Input: part model. Units: mm. Frame: model coordinates. A direction names the side the tool comes from. Give positions to 0.01 mm unless a question says otherwise; leave off trailing zeros. Loops run counter-clockwise (first coordinate to the right, second up) from the corner with the lowest first, then second, coordinate; pieces in that order, holes last. Notation, with made-up numbers: (-36, 46.5) - (-1, 46.5) arc R19 cw to (-1, 72.5) - close; hole circle Ø2 at (76.5, -38). An arc over 180 degrees is marked (long way). One line per item, written item: value.
from build123d import *

# Parameters (mm, degrees)
F0_R     = 63.5
F0_R_2   = 57.15
F0_R_3   = 1.3462
F1_DEPTH = 6.35
F2_START = 3.175
F2_DEPTH = 3.175
F3_SIZE  = 0.635
F4_DEPTH = 1.27


with BuildPart() as f1:
    # F0 (on Top) → F1 (new body)
    with BuildSketch(Plane.XY):
        Circle(F0_R)
        Circle(F0_R_2, mode=Mode.SUBTRACT)
        Circle(F0_R_2)
        with Locations((6.0491874454, -10.4775)):
            Circle(F0_R_3, mode=Mode.SUBTRACT)
        with BuildLine():
            ThreePointArc((-41.4540905122, -2.3213766309), (-39.8240691544, -4.0494939415), (-39.2315905122, -6.35))
            ThreePointArc((-39.2315905122, -6.35), (-46.2945965707, -10.5200213579), (-46.5340905122, -2.3213766309))
            Line((-46.5340905122, -2.3213766309), (-46.5340905122, 2.3213766309))
            ThreePointArc((-46.5340905122, 2.3213766309), (-46.2945965707, 10.5200213579), (-39.2315905122, 6.35))
            ThreePointArc((-39.2315905122, 6.35), (-39.8240691544, 4.0494939415), (-41.4540905122, 2.3213766309))
            Line((-41.4540905122, 2.3213766309), (-41.4540905122, -2.3213766309))
        make_face(mode=Mode.SUBTRACT)
        with Locations((-12.0983748909, 0)):
            Circle(F0_R_3, mode=Mode.SUBTRACT)
        with Locations((6.0491874454, 10.4775)):
            Circle(F0_R_3, mode=Mode.SUBTRACT)
        with BuildLine():
            ThreePointArc((48.7565905122, 6.35), (48.1641118701, 4.0494939415), (46.5340905122, 2.3213766309))
            Line((46.5340905122, 2.3213766309), (46.5340905122, -2.3213766309))
            ThreePointArc((46.5340905122, -2.3213766309), (48.1641118701, -4.0494939415), (48.7565905122, -6.35))
            ThreePointArc((48.7565905122, -6.35), (41.6935844538, -10.5200213579), (41.4540905122, -2.3213766309))
            Line((41.4540905122, -2.3213766309), (41.4540905122, 2.3213766309))
            ThreePointArc((41.4540905122, 2.3213766309), (41.6935844538, 10.5200213579), (48.7565905122, 6.35))
        make_face(mode=Mode.SUBTRACT)
        with BuildLine():
            ThreePointArc((-46.5340905122, -2.3213766309), (-46.2945965707, -10.5200213579), (-39.2315905122, -6.35))
            ThreePointArc((-39.2315905122, -6.35), (-39.8240691544, -4.0494939415), (-41.4540905122, -2.3213766309))
            Line((-41.4540905122, -2.3213766309), (-41.4540905122, -6.35))
            ThreePointArc((-41.4540905122, -6.35), (-43.9940905122, -8.89), (-46.5340905122, -6.35))
            Line((-46.5340905122, -6.35), (-46.5340905122, -2.3213766309))
        make_face()
        with BuildLine():
            ThreePointArc((41.4540905122, 6.35), (43.9940905122, 8.89), (46.5340905122, 6.35))
            Line((46.5340905122, 6.35), (46.5340905122, 2.3213766309))
            ThreePointArc((46.5340905122, 2.3213766309), (48.1641118701, 4.0494939415), (48.7565905122, 6.35))
            ThreePointArc((48.7565905122, 6.35), (41.6935844538, 10.5200213579), (41.4540905122, 2.3213766309))
            Line((41.4540905122, 2.3213766309), (41.4540905122, 6.35))
        make_face()
    extrude(amount=F1_DEPTH)

    # F0 (on Top) → F2 (cut)
    with BuildSketch(Plane.XY.offset(F2_START)):
        with BuildLine():
            ThreePointArc((-46.5340905122, -2.3213766309), (-46.2945965707, -10.5200213579), (-39.2315905122, -6.35))
            ThreePointArc((-39.2315905122, -6.35), (-39.8240691544, -4.0494939415), (-41.4540905122, -2.3213766309))
            Line((-41.4540905122, -2.3213766309), (-41.4540905122, -6.35))
            ThreePointArc((-41.4540905122, -6.35), (-43.9940905122, -8.89), (-46.5340905122, -6.35))
            Line((-46.5340905122, -6.35), (-46.5340905122, -2.3213766309))
        make_face()
        with BuildLine():
            Line((-41.4540905122, -6.35), (-41.4540905122, -2.3213766309))
            ThreePointArc((-41.4540905122, -2.3213766309), (-43.9940905122, -1.5875), (-46.5340905122, -2.3213766309))
            Line((-46.5340905122, -2.3213766309), (-46.5340905122, -6.35))
            ThreePointArc((-46.5340905122, -6.35), (-43.9940905122, -3.81), (-41.4540905122, -6.35))
        make_face()
        with BuildLine():
            Line((46.5340905122, 2.3213766309), (46.5340905122, 6.35))
            ThreePointArc((46.5340905122, 6.35), (43.9940905122, 3.81), (41.4540905122, 6.35))
            Line((41.4540905122, 6.35), (41.4540905122, 2.3213766309))
            ThreePointArc((41.4540905122, 2.3213766309), (43.9940905122, 1.5875), (46.5340905122, 2.3213766309))
        make_face()
        with BuildLine():
            ThreePointArc((41.4540905122, 6.35), (43.9940905122, 8.89), (46.5340905122, 6.35))
            Line((46.5340905122, 6.35), (46.5340905122, 2.3213766309))
            ThreePointArc((46.5340905122, 2.3213766309), (48.1641118701, 4.0494939415), (48.7565905122, 6.35))
            ThreePointArc((48.7565905122, 6.35), (41.6935844538, 10.5200213579), (41.4540905122, 2.3213766309))
            Line((41.4540905122, 2.3213766309), (41.4540905122, 6.35))
        make_face()
    extrude(amount=F2_DEPTH, mode=Mode.SUBTRACT)

    # F3
    f3_edges = [f1.edges().sort_by_distance(p)[0] for p in [
        (-63.5, 0, 6.35),
    ]]
    chamfer(f3_edges, length=F3_SIZE)

    # F0 (on Top) → F4 (cut)
    with BuildSketch(Plane.XY):
        Circle(F0_R_2)
        with Locations((6.0491874454, -10.4775)):
            Circle(F0_R_3, mode=Mode.SUBTRACT)
        with BuildLine():
            ThreePointArc((-41.4540905122, -2.3213766309), (-39.8240691544, -4.0494939415), (-39.2315905122, -6.35))
            ThreePointArc((-39.2315905122, -6.35), (-46.2945965707, -10.5200213579), (-46.5340905122, -2.3213766309))
            Line((-46.5340905122, -2.3213766309), (-46.5340905122, 2.3213766309))
            ThreePointArc((-46.5340905122, 2.3213766309), (-46.2945965707, 10.5200213579), (-39.2315905122, 6.35))
            ThreePointArc((-39.2315905122, 6.35), (-39.8240691544, 4.0494939415), (-41.4540905122, 2.3213766309))
            Line((-41.4540905122, 2.3213766309), (-41.4540905122, -2.3213766309))
        make_face(mode=Mode.SUBTRACT)
        with Locations((-12.0983748909, 0)):
            Circle(F0_R_3, mode=Mode.SUBTRACT)
        with Locations((6.0491874454, 10.4775)):
            Circle(F0_R_3, mode=Mode.SUBTRACT)
        with BuildLine():
            ThreePointArc((48.7565905122, 6.35), (48.1641118701, 4.0494939415), (46.5340905122, 2.3213766309))
            Line((46.5340905122, 2.3213766309), (46.5340905122, -2.3213766309))
            ThreePointArc((46.5340905122, -2.3213766309), (48.1641118701, -4.0494939415), (48.7565905122, -6.35))
            ThreePointArc((48.7565905122, -6.35), (41.6935844538, -10.5200213579), (41.4540905122, -2.3213766309))
            Line((41.4540905122, -2.3213766309), (41.4540905122, 2.3213766309))
            ThreePointArc((41.4540905122, 2.3213766309), (41.6935844538, 10.5200213579), (48.7565905122, 6.35))
        make_face(mode=Mode.SUBTRACT)
        with BuildLine():
            ThreePointArc((-46.5340905122, -2.3213766309), (-46.2945965707, -10.5200213579), (-39.2315905122, -6.35))
            ThreePointArc((-39.2315905122, -6.35), (-39.8240691544, -4.0494939415), (-41.4540905122, -2.3213766309))
            Line((-41.4540905122, -2.3213766309), (-41.4540905122, -6.35))
            ThreePointArc((-41.4540905122, -6.35), (-43.9940905122, -8.89), (-46.5340905122, -6.35))
            Line((-46.5340905122, -6.35), (-46.5340905122, -2.3213766309))
        make_face()
        with BuildLine():
            ThreePointArc((41.4540905122, 6.35), (43.9940905122, 8.89), (46.5340905122, 6.35))
            Line((46.5340905122, 6.35), (46.5340905122, 2.3213766309))
            ThreePointArc((46.5340905122, 2.3213766309), (48.1641118701, 4.0494939415), (48.7565905122, 6.35))
            ThreePointArc((48.7565905122, 6.35), (41.6935844538, 10.5200213579), (41.4540905122, 2.3213766309))
            Line((41.4540905122, 2.3213766309), (41.4540905122, 6.35))
        make_face()
    extrude(amount=F4_DEPTH, mode=Mode.SUBTRACT)


solid = f1.part
Item 1: Section A-A, the plane x = 0. Output: boundary loops of the cut face in (y, z) (3 decimals), and give its area (3 significant figures).
Verdict:
outline: (-63.5, 0) - (-57.15, 0) - (-57.15, 1.27) - (57.15, 1.27) - (57.15, 0) - (63.5, 0) - (63.5, 5.715) - (62.865, 6.35) - (-62.865, 6.35) - (-63.5, 5.715) - close
area: 661 mm^2
Item 2: Material intervals for L1, parallel to X at y = -9, z = 5.25; L2, parallel to Z at x = -12.5, y = -2.5; L3, parallel to X at y = 3, z = 4.5, sorted ascending.
Verdict:
L1: x = -62.86 to -47.95, -40.04 to 40.04, 47.95 to 62.86
L2: z = 1.27 to 6.35
L3: x = -63.43 to -47.38, -40.61 to 40.61, 47.38 to 63.43
Item 3: Access query for faces 4 (the face through (-57.095, 2.513, 0.626)), 5 (the face through (-44, -10, 3.175)), 6 (the face through (46.534, 1, 3)). Directions: +Z, -Z, +X, -X, +Y, -Y. A direction counts if a zero-diameter tool reaches every point of the face in a straight line with its end or side. Return the directions, or none.
Verdict:
face 4: -Z
face 5: +Z
face 6: +Z, -Z
Item 4: Section B-B, the plane z = 4.75. Count the separate pieces of the cut face and the enclosed holes in it, and give its area (3 significant figures).
Verdict:
separate pieces: 1
enclosed holes: 5
area: 12,300 mm^2
Item 5: Pin query (flat end, axial travel): P1, Ø2, axis at x = -12.1, y = 0, coming from the +Z side; P2, Ø3, axis at y = 21, z = 4.5, coming from the -X side; P3, Ø5.5, axis at x = -43.99, y = -6.35, coming from the +Z side (3 decimals); P4, Ø1, axis at x = -13.5, z = 3.5, coming from the +Y side. Return the tip coordinate at first contact, or that it passes through.
Verdict:
P1: passes through
P2: stops at x = -60.43
P3: stops at z = 3.175
P4: stops at y = 62.16
Item 6: Draft query along X for faces 1 (the face through (-41.454, -1, 3)), 2 (the face through (-13.77, -61.99, 2.82)), 3 (the face through (-57, 10, 0)). Return one class per face: pulls with the +X half, pulls with the -X half, needs draft (parallel to the pull), parting line crosses it, or undercut.
Verdict:
face 1: undercut
face 2: parting line crosses it
face 3: needs draft
